Work out the finished part from the listing and answer in its coordinate system (mm). A direction names the side the tool comes from. Coordinates: 2 decimals unless noted, no trailing zeros. Loops run counter-clockwise (first coordinate to the right, second up) from the corner with the lowest first, then second, coordinate; pieces in that order, holes last. Notation, with made-up numbers: (48, 39) - (83, 39) arc R33 ccw to (83, 69) - close; hole circle Ø9 at (87, -15). An arc over 180 degrees is marked (long way). Write each question's results on one line, items separated by ' | '. Start each with the question number.
1. Find the intervals of material crossed by line 1 along Z through (x, y) = (17.75, -15.24); line 2 along Z through (x, y) = (4.5, -36); line 3 along Y through (x, z) = (15, -58), in increasing order. Write a range as [from, to].
2. Which of the six approach directions +Z, -Z, +X, -X, +Y, -Y give full straight-line access (tool end or side, diameter ignored) to faces 1 (the cylindrical face through (17.91, -2.68, -60.11)), 2 (the cylindrical face through (1.449, -1.528, 12.878)), 3 (the cylindrical face through (19.14, -19.92, 22.07))?
3. A cutting plane is placed at B-B on y = -12.7. Determine the outline of the cut face in (x, z).
4. Each of these flat-tipped pins is pushed along its axis until it touches: P1, Ø5, axis at x = 10, z = -43.5, coming from the -Y side; P2, Ø11.5, axis at y = -15.24, z = 17.78, coming from the +X side; P3, Ø1.5, axis at x = 8, z = -94.5, coming from the -Y side. Where does it stop, or does it pass through?
5. A cutting plane is placed at A-A on z = 17.78. Determine the outline of the cut face in (x, y), then the cut area to 3 significant figures.
6. Determine the mould class of faces 4 (the flat face through (12.7, -15, 18)), 5 (the flat face through (13, -13, -127)), 6 (the cylindrical face through (12.878, -1.449, 23.872)), 7 (the flat face through (13, -50.8, 13)) for opening direction Z: released by +Z, released by -Z, zero draft, split by the parting line, or undercut.
7. A cutting plane is placed at D-D on z = -3.5. Determine the outline of the cut face in (x, y).
8. A cutting plane is placed at C-C on y = -35.5. Determine the outline of the cut face in (x, z), then the cut area to 3 significant figures.
from build123d import *

# Parameters (mm, degrees)
F0_W     = 25.4
F0_H     = 50.8
F1_DEPTH = 25.4
F2_R     = 5.08
F3_R     = 11.294714
F4_DEPTH = 127
F5_SIZE  = 5.08
F6_R     = 6.35
F7_DEPTH = 12.7


with BuildPart() as f1:
    # F0 (on Top) → F1 (new body)
    with BuildSketch(Plane.XY):
        with Locations((12.7, -25.4)):
            Rectangle(F0_W, F0_H)
    extrude(amount=F1_DEPTH)

    # F2
    f2_edges = [f1.edges().sort_by_distance(p)[0] for p in [
        (12.7, 0, 25.4),
        (25.4, 0, 12.7),
        (0, 0, 12.7),
    ]]
    fillet(f2_edges, radius=F2_R)

    # F3 (on face) → F4 (join)
    with BuildSketch(Plane(origin=(0, 0, 0), x_dir=(1, 0, 0), z_dir=(0, 0, -1))):
        with Locations((12.7, 12.7)):
            Circle(F3_R)
    extrude(amount=F4_DEPTH)

    # F5
    f5_edges = [f1.edges().sort_by_distance(p)[0] for p in [
        (1.405286, -12.7, -127),
    ]]
    chamfer(f5_edges, length=F5_SIZE)

    # F6 (on face) → F7 (cut)
    with BuildSketch(Plane.YZ.offset(25.4)):
        with Locations((-15.24, 17.78)):
            Circle(F6_R)
    extrude(amount=-F7_DEPTH, mode=Mode.SUBTRACT)


solid = f1.part
Values:
1) line 1: [-127, 11.43], [24.13, 25.4] | line 2: [0, 25.4] | line 3: [-23.76, -1.64]
2) face 1: -Z | face 2: +Z, -Z, -X, +Y | face 3: +X
3) outline: (0, 0) - (1.41, 0) - (1.41, -121.92) - (6.49, -127) - (18.91, -127) - (23.99, -121.92) - (23.99, 0) - (25.4, 0) - (25.4, 11.96) - (12.7, 11.96) - (12.7, 23.6) - (25.4, 23.6) - (25.4, 25.4) - (0, 25.4) - close
4) P1: y = -23.99 | P2: x = 12.7 | P3: y = -23.28
5) outline: (0, -50.8) - (25.4, -50.8) - (25.4, -21.59) - (12.7, -21.59) - (12.7, -8.89) - (25.4, -8.89) - (25.4, -5.08) arc R5.08 ccw to (20.32, 0) - (5.08, 0) arc R5.08 ccw to (0, -5.08) - close | area: 1,120 mm^2
6) face 4: undercut | face 5: released by -Z | face 6: released by +Z | face 7: zero draft
7) outline: circle Ø22.59 at (12.7, -12.7)
8) outline: (0, 0) - (25.4, 0) - (25.4, 25.4) - (0, 25.4) - close | area: 645 mm^2
